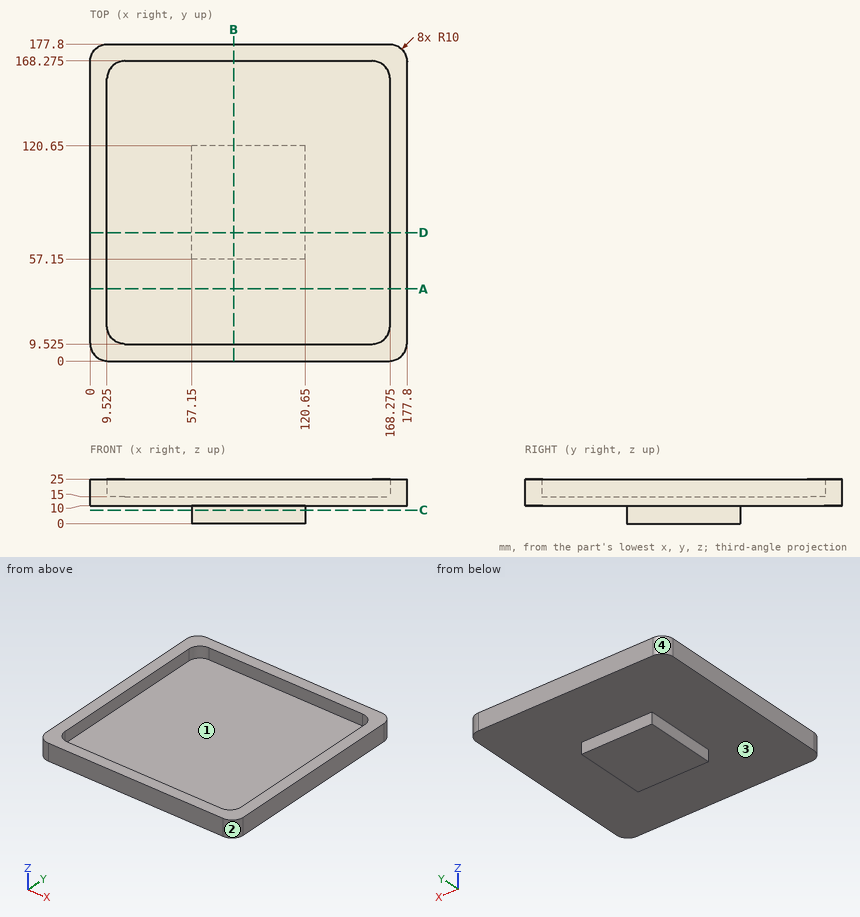
Job drawing, mm, ordinate dimensions from the low corner. One solid piece. Give positions to 0.01 mm unless a question says otherwise; leave off trailing zeros. Write each loop counter-clockwise with the first axis right and the second up, starting at its lowest first coordinate (ties: lowest second). Pieces come first, ordered by that corner, then holes. Notation, with made-up numbers: M 68.25,10.5 L 79.25,10.5 A25 cw 79.25,32.5 Z; hole C -14,-27.75 d3. An arc over 180 degrees is marked long. Put each result on its own line as item: value. Start each with the question number.
(1) Band-saw the part on B-B, the plane x = 80.5. Write the cut outline in (y, z) (3 decimals).
(2) Probe L1, parallel to X at y = 40.5, z = 20 (3 decimals); L2, parallel to X at y = 159, z = 16.5. List the from-to ranges inside material, lowest first.
(3) Band-saw the part on A-A, the plane y = 40.5. Write the cut outline in (x, z) (3 decimals).
(4) Flat gauge pins, fed straight in: pin 1 Ø5 at (y, z) = (94, 3) entering from +X; pin 2 Ø8 at (x, z) = (61, 3) entering from +Y; pin 3 Ø1.5 at (y, z) = (19, 8.5) entering from +X; pin 4 Ø3 at (x, z) = (97, 6.5) entering from -Y. Where does each tip first touch, or does it go through?
(5) Mould opens along X. For the marked faces 1, 2, 3 and 4 say: +X half, -X half, draft (parallel to the pull), parting line (faces both ways), or undercut.
(6) Band-saw the part on C-C, the plane z = 7.5. Write the cut outline in (x, y), and give its area (3 significant figures).
Response values:
1. outline: M 0,10 L 57.15,10 L 57.15,0 L 120.65,0 L 120.65,10 L 177.8,10 L 177.8,25 L 168.275,25 L 168.275,15 L 9.525,15 L 9.525,25 L 0,25 Z
2. L1: x = 0 to 9.525, 168.275 to 177.8
2. L2: x = 0 to 9.55, 168.25 to 177.8
3. outline: M 0,10 L 177.8,10 L 177.8,25 L 168.275,25 L 168.275,15 L 9.525,15 L 9.525,25 L 0,25 Z
4. pin 1: stops at x = 120.65
4. pin 2: stops at y = 120.65
4. pin 3: passes through
4. pin 4: stops at y = 57.15
5. face 1: undercut
5. face 2: +X half
5. face 3: draft
5. face 4: -X half
6. outline: M 57.15,57.15 L 120.65,57.15 L 120.65,120.65 L 57.15,120.65 Z
6. area: 4,030 mm2
